Input: part model. Units: mm. Frame: model coordinates. Face numbers are marked on the shaded views. A direction names the side the tool comes from. Round coordinates to 2 decimals unless told otherwise and drop trailing zeros. Loops run counter-clockwise (first coordinate to the right, second up) from the corner with the lowest first, then second, coordinate; pieces in that order, holes last.
1) First-contact query: pin 1 (3 mm diameter, centred on y = -5.5, z = 10.5, fed in from +X); pin 2 (4 mm diameter, centred on x = 3.5, y = 5.5, fed in from -Z); pin 3 (3 mm diameter, centred on y = -1.5, z = 2, fed in from -X); pin 4 (5 mm diameter, centred on x = 4, z = 5.5, fed in from +Y). Flat tips, straight axial feed; report the tip coordinate or a pass-through.
2) Section A-A, the plane z = 5. Return loops of the section in (x, y).
3) Draft query along Y for the marked faces 1, 2 and 3. Return one class per face: pulls with the +Y half, pulls with the -Y half, needs draft (parallel to the pull), parting line crosses it, or undercut.
4) Access query for the marked faces 4 and 5. Directions: +Z, -Z, +X, -X, +Y, -Y. A direction counts if a zero-diameter tool reaches every point of the face in a straight line with its end or side. Return the directions, or none.
5) Section B-B, the plane z = 12.75. State how many separate pieces and enclosed holes the cut face has, and give its area (3 significant figures).
6) Ray query, line 1 along Y through (x, z) = (2.5, 12.75); line 2 along Z through (x, y) = (-2.5, 5); line 3 along Z through (x, y) = (-5.75, 3.25). Return the intervals inside material, ascending.
from build123d import *

# Parameters (mm, degrees)
SKETCH1_R           = 7
BOSS_EXTRUDE1_DEPTH = 14
SKETCH2_OUTSIDE_W   = 20.85
SKETCH2_OUTSIDE_H   = 20.85
SKETCH2_OUTSIDE_R   = 6
CUT_EXTRUDE1_DEPTH  = 10
SKETCH3_R           = 5.5
CUT_EXTRUDE2_DEPTH  = 1.5
CUT_EXTRUDE2_TAPER  = 45
SKETCH4_R           = 4
CUT_EXTRUDE3_DEPTH  = 12.5
SKETCH5_R           = 4
BOSS_EXTRUDE3_DEPTH = 12.5


with BuildPart() as part:
    # Sketch1 → Boss-Extrude1 (new body)
    with BuildSketch(Plane.XY):
        Circle(SKETCH1_R)
    extrude(amount=BOSS_EXTRUDE1_DEPTH)

    # Sketch2 outside → Cut-Extrude1 (cut)
    with BuildSketch(Plane(origin=(0, 0, 0), x_dir=(-1, 0, 0), z_dir=(0, 0, -1))):
        Rectangle(SKETCH2_OUTSIDE_W, SKETCH2_OUTSIDE_H)
        Circle(SKETCH2_OUTSIDE_R, mode=Mode.SUBTRACT)
    extrude(amount=-CUT_EXTRUDE1_DEPTH, mode=Mode.SUBTRACT)

    # Sketch3 → Cut-Extrude2 (cut)
    with BuildSketch(Plane.XY.offset(14)):
        Circle(SKETCH3_R)
    extrude(amount=-CUT_EXTRUDE2_DEPTH, taper=CUT_EXTRUDE2_TAPER, mode=Mode.SUBTRACT)

    # Sketch4 → Cut-Extrude3 (cut)
    with BuildSketch(Plane.XY.offset(12.5)):
        Circle(SKETCH4_R)
    extrude(amount=-CUT_EXTRUDE3_DEPTH, mode=Mode.SUBTRACT)



with BuildPart() as body_2:
    # Sketch5 → Boss-Extrude3 (new body)
    with BuildSketch(Plane(origin=(0, 0, 0), x_dir=(-1, 0, 0), z_dir=(0, 0, -1))):
        Circle(SKETCH5_R)
    extrude(amount=-BOSS_EXTRUDE3_DEPTH)


with BuildPart() as part_1:
    add(part.part)

    add(body_2.part)  # Revolve1 merges body 2
    # Sketch6 → Revolve1 (revolve)
    with BuildSketch(Plane(origin=(0, 0, 0), x_dir=(1, 0, 0), z_dir=(0, 1, 0))):
        with BuildLine():
            Line((-4, -12.5), (0, -12.5))
            Line((0, -12.5), (0, -14))
            ThreePointArc((0, -14), (-2.168263504, -13.698702678), (-4, -12.5))
        make_face()
    revolve(axis=Axis((0, 0, 12.5), (0, 0, 1)))


solid = part_1.part
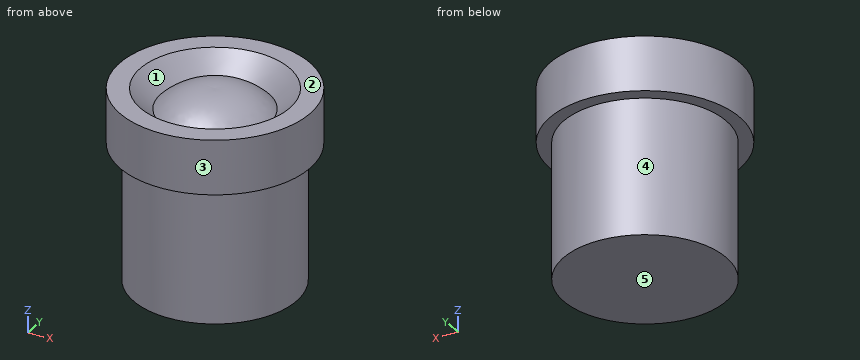
Final values:
1. pin 1: stops at x = 5.74
1. pin 2: stops at z = 0
1. pin 3: stops at x = -6
1. pin 4: stops at y = 5.81
2. outline: circle Ø12 at (0, 0)
3. face 1: undercut
3. face 2: needs draft
3. face 3: parting line crosses it
4. face 4: -Z
4. face 5: -Z, +X, -X, +Y, -Y
5. separate pieces: 2
5. enclosed holes: 1
5. area: 141 mm2
6. line 1: y = -6.54 to -3.44, -2.78 to 2.78, 3.44 to 6.54
6. line 2: z = 0 to 14
6. line 3: z = 10 to 14
